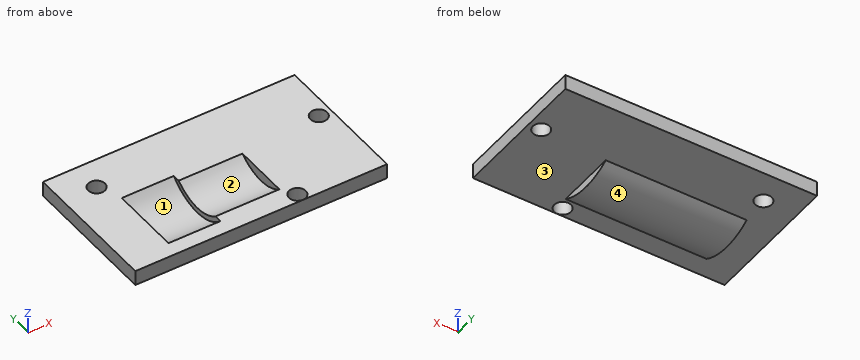
from build123d import *

# Parameters (mm, degrees)
SKETCH1_W            = 15
SKETCH1_H            = 8.3
SKETCH1_R            = 0.5
FRONT_FACE_EXT_DEPTH = 0.9
BOSS_EXTRUDE1_START  = -0.3
BOSS_EXTRUDE1_DEPTH  = 8.4
CUT_EXTRUDE5_START   = -1
CUT_EXTRUDE5_DEPTH   = 3.1
CUT_EXTRUDE6_DEPTH   = 3.8


with BuildPart() as part:
    # Sketch1 → Front Face Ext (new body)
    with BuildSketch(Plane.XY):
        Rectangle(SKETCH1_W, SKETCH1_H)
        with Locations((-5.5, 2.35)):
            Circle(SKETCH1_R, mode=Mode.SUBTRACT)
        with Locations((6.75, 0.85)):
            Circle(SKETCH1_R, mode=Mode.SUBTRACT)
        with Locations((2.498361092, -3.64)):
            Circle(SKETCH1_R, mode=Mode.SUBTRACT)
    extrude(amount=FRONT_FACE_EXT_DEPTH)

    # Sketch3 → Boss-Extrude1 (add)
    with BuildSketch(Plane.ZY.offset(5.93).offset(BOSS_EXTRUDE1_START)):
        with BuildLine():
            Line((0, 0.65), (0, -2.96))
            ThreePointArc((0, -2.96), (-0.501337798, -1.155), (0, 0.65))
        make_face()
    extrude(amount=-BOSS_EXTRUDE1_DEPTH)

    # Sketch4 → Cut-Extrude5 (cut)
    with BuildSketch(Plane.ZY.offset(5.93).offset(CUT_EXTRUDE5_START)):
        with BuildLine():
            Line((0.9, 0.945), (0.9, -3.255))
            ThreePointArc((0.9, -3.255), (0, -1.155), (0.9, 0.945))
        make_face()
    extrude(amount=-CUT_EXTRUDE5_DEPTH, mode=Mode.SUBTRACT)

    # Sketch6 → Cut-Extrude6 (cut)
    with BuildSketch(Plane.ZY.offset(1.83)):
        with BuildLine():
            Line((0.9, 0.506324773), (0.9, -2.816324773))
            ThreePointArc((0.9, -2.816324773), (0.3, -1.155), (0.9, 0.506324773))
        make_face()
    extrude(amount=-CUT_EXTRUDE6_DEPTH, mode=Mode.SUBTRACT)


solid = part.part
Model file for the job. Use its own axes, mm. Face numbers are marked on the shaded views. Give positions to 0.01 mm unless a question says otherwise; leave off trailing zeros. Order: outer loops, then holes, each group sorted by start corner. A loop starts at its lowest first (then second) coordinate and runs counter-clockwise, first axis right, second up. Notation, with made-up numbers: (50.5, -6.75) - (101.5, -6.75) arc R29 ccw to (101.5, 20.25) - close; hole circle Ø10 at (9, 27). An arc over 180 degrees is marked (long way). Write item = value, one per line. Start each with the question number.
1. Two-plate mould, pull along Y, no slides. Class the marked faces 1, 2, 3 and 4: pulls with the +Y half, pulls with the -Y half, needs draft (parallel to the pull), parting line crosses it, or undercut.
2. Drop flat-ended pins along their axis: P1, Ø2.5, axis at x = -1.5, y = 1, coming from the -Z side; P2, Ø3, axis at x = 6, y = 3, coming from the -Z side. Give the stop position or say it passes through.
3. Cut at C-C, the plane x = -4.5. List the corners of the cut face in (y, z) (3 decimals).
4. Cut at A-A, the plane y = -3.64. List the corners of the cut face in (x, z), and give its area (3 significant figures).
5. Cut at D-D, the plane z = 0.7. List the corners of the cut face in (x, y), and give its area (3 significant figures).
6. Probe line 1 along X through (y, z) = (-2.25, 0.3); line 2 along Y through (x, z) = (-5.5, 0.75); line 3 along Y through (x, z) = (6.75, 0.5). List the from-to ranges inside material, lowest first.
7. Cut at B-B, the plane x = 6.75. List the corners of the cut face in (y, z).
Taken from the geometry:
q1.face_1 = undercut
q1.face_2 = undercut
q1.face_3 = needs draft
q1.face_4 = parting line crosses it
q2.P1 = -0.38
q2.P2 = 0
q3.outline = (-4.15, 0) - (-2.96, 0) arc R3.5 ccw to (0.65, 0) - (4.15, 0) - (4.15, 0.9) - (0.945, 0.9) arc R2.9 cw to (-3.255, 0.9) - (-4.15, 0.9) - close
q4.outline = (-7.5, 0) - (2, 0) - (2, 0.9) - (-7.5, 0.9) - close; (3, 0) - (7.5, 0) - (7.5, 0.9) - (3, 0.9) - close
q4.area = 12.6 mm²
q5.outline = (-7.5, -4.15) - (7.5, -4.15) - (7.5, 4.15) - (-7.5, 4.15) - close; hole circle Ø1 at (-5.5, 2.35); hole (-4.93, -3.04) - (-1.83, -3.04) - (-1.83, -2.54) - (1.97, -2.54) - (1.97, 0.23) - (-1.83, 0.23) - (-1.83, 0.73) - (-4.93, 0.73) - close; hole circle Ø1 at (2.5, -3.64); hole circle Ø1 at (6.75, 0.85)
q5.area = 99.9 mm²
q6.line_1 = -7.5 to -4.93, -1.83 to 7.5
q6.line_2 = -4.15 to 1.85, 2.85 to 4.15
q6.line_3 = -4.15 to 0.35, 1.35 to 4.15
q7.outline = (-4.15, 0) - (0.35, 0) - (0.35, 0.9) - (-4.15, 0.9) - close; (1.35, 0) - (4.15, 0) - (4.15, 0.9) - (1.35, 0.9) - close
